Answer from the drawing. Dimensions are ordinates in mm from the lowest x, y and z of the part. A direction names the side the tool comes from. Round coordinates to 2 decimals unless told otherwise and drop trailing zeros. Write each loop counter-clockwise with the first axis right and the second up, starting at its lowest first coordinate (ties: lowest second). Pieces come first, ordered by that corner, then holes. Notation, with made-up numbers: (-6, 51) - (3, 51) arc R22 ccw to (3, 57) - close; hole circle Ø8 at (-24, 68.25). An arc over 180 degrees is marked (long way). Use a Markdown table: item, result. Add a question column.
1) A tool of negligible diameter and unlimited length cuts with its end or side. For the marked faces 1 and 2, from which of +Z, -Z, +X, -X, +Y, -Y can it reach the whole face along a straight path? Write none if from no direction.
2) A cutting plane is placed at C-C (y = 14). Give the vertices of the cut face in (x, z).
3) Find the intervals of material crossed by probe 1 along Y at (x, z) = (21.5, 11.5); probe 2 along X at (y, z) = (10.75, 5); probe 3 along Y at (x, z) = (10, 23), in increasing order. Write a range as from..to.
4) A cutting plane is placed at B-B (x = 3). Give the vertices of the cut face in (y, z).
5) A cutting plane is placed at A-A (z = 7.75). Give the vertices of the cut face in (x, y), then the cut area to 3 significant figures.
6) A cutting plane is placed at D-D (z = 3.25). Give the vertices of the cut face in (x, y).
7) Each of these flat-tipped pins is pushed along its axis until it touches: P1, Ø6.5, axis at y = 5.5, z = 6.5, coming from the +X side; P2, Ø5, axis at x = 28.5, y = 9.5, coming from the -Z side; P3, Ø14, axis at x = 31, z = 3, coming from the -Y side. Where does it stop, or does it pass through?
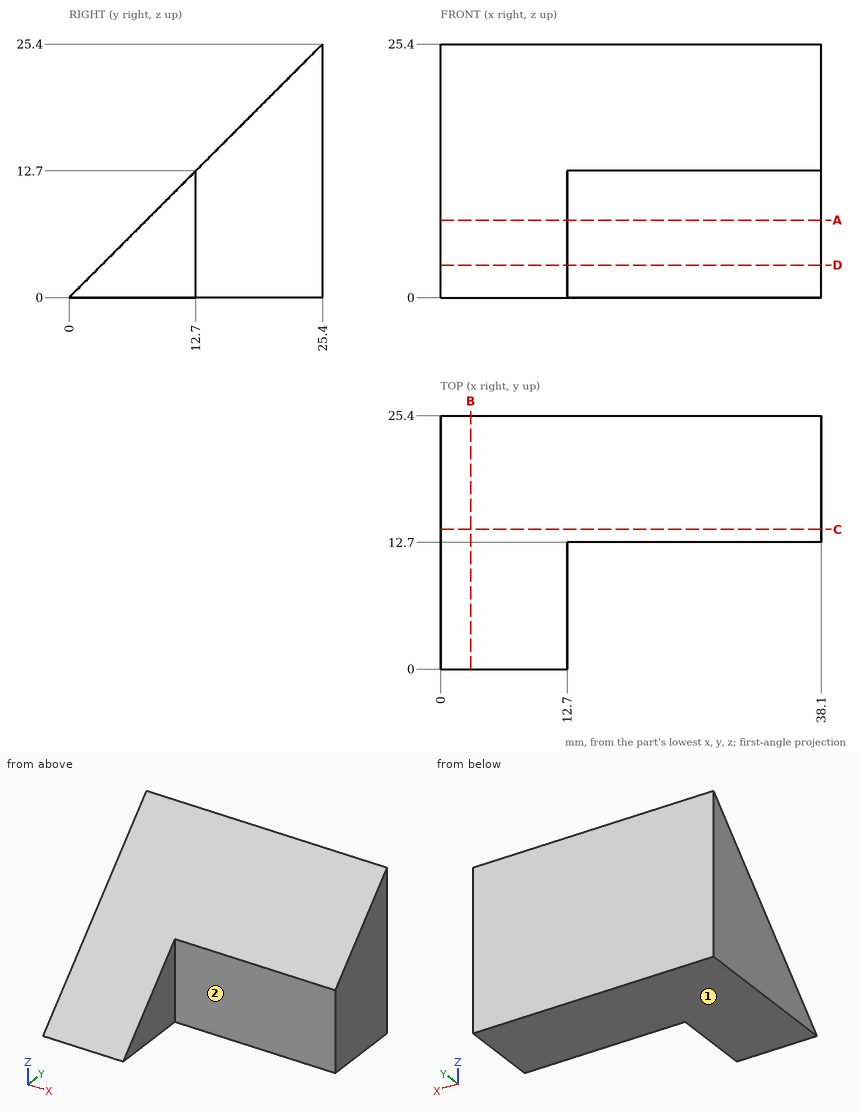
Entries:
| question | item | result |
|---|---|---|
| 1 | face 1 | -Z, +X, -X, +Y, -Y |
| 1 | face 2 | +Z, -Z, +X, -Y |
| 2 | outline | (0, 0) - (38.1, 0) - (38.1, 14) - (0, 14) - close |
| 3 | probe 1 | y = 12.7..25.4 |
| 3 | probe 2 | x = 0..12.7 |
| 3 | probe 3 | y = 23..25.4 |
| 4 | outline | (0, 0) - (25.4, 0) - (25.4, 25.4) - close |
| 5 | outline | (0, 7.75) - (12.7, 7.75) - (12.7, 12.7) - (38.1, 12.7) - (38.1, 25.4) - (0, 25.4) - close |
| 5 | area | 547 mm² |
| 6 | outline | (0, 3.25) - (12.7, 3.25) - (12.7, 12.7) - (38.1, 12.7) - (38.1, 25.4) - (0, 25.4) - close |
| 7 | P1 | stops at x = 12.7 |
| 7 | P2 | passes through |
| 7 | P3 | stops at y = 12.7 |
